Verification items for the finished model (mm, model axes). A direction names the side the tool comes from. Round coordinates to 2 decimals unless told otherwise and drop trailing zeros. Write each loop counter-clockwise with the first axis right and the second up, starting at its lowest first coordinate (ties: lowest second). Pieces come first, ordered by that corner, then holes.
Autodesk Inventor part; units mm, degrees
ref_plane "YZ Plane" through (0, 0, 0) normal (1, 0, 0) x (0, 1, 0)
ref_plane "XZ Plane" through (0, 0, 0) normal (0, 1, 0) x (-1, 0, 0)
ref_plane "XY Plane" through (0, 0, 0) normal (0, 0, 1) x (1, 0, 0)
ref_plane "Work Plane5" through (0, 3, 0) normal (0, 1, 0) x (1, 0, 0)
ref_plane "Work Plane2" through (0, 0, 0) normal (0, -1, 0) x (1, 0, 0)
ref_plane "Work Plane1" through (0, 3, 0) normal (0, 1, 0) x (1, 0, 0)
ref_plane "Work Plane7" through (0, 3, 0) normal (0, -1, 0) x (1, 0, 0)
sketch "Sketch77" plane through (0, 3, 0) normal (0, -1, 0) x (1, 0, 0)
  circle A0 centre (16, 0) radius 17.5
  point P0 (0, 0)
  dimension "d219" = 35
ref_plane "Work Plane6" through (0, 3, 0) normal (0, -1, 0) x (1, 0, 0)
sketch "Sketch78" plane through (0, 3, 0) normal (0, -1, 0) x (1, 0, 0)
  line L0 (45, -30) -> (-13, -30)
  line L1 (-13, -30) -> (-13, 30)
  line L2 (-13, 30) -> (45, 30)
  line L3 (45, 30) -> (45, -30)
  line L4 (45, -30) -> (-13, 30) construction
  line L5 (-13, -30) -> (45, 30) construction
  point P0 (0, 0)
  point P1 (16, 0)
  dimension "d220" = 58
  dimension "d221" = 60
extrude "Extrusion53" add sketch "Sketch78" against normal blind 3
extrude "Extrusion54" cut sketch "Sketch77" against normal blind 3
ref_plane "Work Plane9" through (0, 3, 0) normal (0, -1, 0) x (1, 0, 0)
sketch "Sketch81" plane through (0, 3, 0) normal (0, -1, 0) x (1, 0, 0)
  circle A0 centre (33.5, -25) radius 2.7
  line L0 (-13, -30) -> (45, -30)
  line L1 (45, -30) -> (45, 30)
  circle A1 centre (16, -25) radius 2.7
  circle A2 centre (-1.5, -25) radius 2.7
  circle A3 centre (-6.5, -8) radius 2.7
  circle A4 centre (-6.5, 8) radius 2.7
  circle A5 centre (-1.5, 25) radius 2.7
  circle A6 centre (16, 25) radius 2.7
  circle A7 centre (33.5, 25) radius 2.7
  point P0 (0, 0)
  dimension "mag_D" = 5.4
  dimension "d232" = 5
  dimension "d233" = 11.5
  dimension "d234" = 5.4
  dimension "d235" = 17.5
  dimension "d236" = 5.4
  dimension "d237" = 17.5
  dimension "d238" = 5.4
  dimension "d239" = 5
  dimension "d240" = 17
  dimension "d241" = 5.4
  dimension "d242" = 16
  dimension "d243" = 5.4
  dimension "d244" = 17
  dimension "d245" = 5.4
  dimension "d246" = 17.5
  dimension "d247" = 5.4
  dimension "d248" = 17.5
  dimension "d249" = 5
extrude "Extrusion56" cut sketch "Sketch81" against normal blind 30
ref_plane "Work Plane8" through (0, 3, 0) normal (0, -1, 0) x (1, 0, 0)
sketch "Sketch83" plane through (0, 3, 0) normal (0, -1, 0) x (1, 0, 0)
  circle A0 centre (-6.5, -8) radius 2.7
  line L0 (-9.1417, -2.4) -> (-9.1417, 2.4)
  line L1 (-9.1417, 2.4) -> (-4.9848, 0)
  line L2 (-4.9848, 0) -> (-9.1417, -2.4)
  point P0 (0, 0)
  point P1 (-9.1417, -8.5581)
  point P2 (-7.756, 0)
  dimension "d253" = 4.8
extrude "Extrusion57" add sketch "Sketch83" along normal blind 4.5 contours L0 L1 L2
sketch "Sketch84" plane through (0, 6, 0) normal (0, 1, 0) x (1, 0, 0)
  point P0 (0, 0)
equation "\"d234\" = mag_D"
equation "\"d236\" = mag_D"
equation "\"d237\" = d235"
equation "\"d238\" = mag_D"
equation "\"d241\" = mag_D"
equation "\"d243\" = mag_D"
equation "\"d244\" = d240"
equation "\"d245\" = mag_D"
equation "\"d246\" = d235"
equation "\"d247\" = mag_D"
equation "\"d248\" = d235"
equation "\"d249\" = d239"
properties part number "liquid_port_v03_printtest"
Q1. Depth check by flat-ended pin: P1, Ø7, axis at x = 33.5, z = 25, coming from the -Y side. Enter the tip coordinate at first touch or a pass-through.
Recorded:
P1: stops at y = 3
Q2. Material ranges on line 1 along Z through (x, y) = (16, 3.7); line 2 along Z through (x, y) = (-6.5, 3.7); line 3 along X through (y, z) = (4, 27), recorded low to high.
Recorded:
line 1: z = -30 to -27.7, -22.3 to -17.5, 17.5 to 22.3, 27.7 to 30
line 2: z = -30 to -10.7, -5.3 to 5.3, 10.7 to 30
line 3: x = -13 to -3.31, 0.31 to 14.19, 17.81 to 31.69, 35.31 to 45
Q3. Release check for a two-part mould opening along X. For faces 4 (the flat face through (3, 3, 14)), 5 (the cylindrical face through (-1.851, 4.479, -22.323)), 6 (the flat face through (-13, 4, 0)), 7 (the cylindrical face through (-1.851, 4.479, 27.677)) record: released by +X, released by -X, zero draft, split by the parting line, or undercut.
Recorded:
face 4: zero draft
face 5: undercut
face 6: released by -X
face 7: undercut
Q4. Tool access check on faces 1 (the flat face through (-7.03, 0.78, -1.18)), 2 (the flat face through (-9.142, 1, 0)), 3 (the flat face through (-7.092, 0.781, 1.217)). Record the directions out of +Z, -Z, +X, -X, +Y, -Y that give a thin tool (end or side, any length) a straight path to the whole face; none if there is none.
Recorded:
face 1: -Z, +X, -Y
face 2: +Z, -Z, -X, -Y
face 3: +Z, +X, -Y
Q5. Sectioned sample at B-B (y = 5). Give the number of separate pieces and of enclosed holes in the cut face, plus the area to 3 significant figures.
Recorded:
separate pieces: 1
enclosed holes: 9
area: 2,330 mm2
Q6. Sectioned sample at A-A (z = 25). Enter the section's corners in (x, y), plus the area to 3 significant figures.
Recorded:
outline: (-13, 3) - (-4.2, 3) - (-4.2, 6) - (-13, 6) - close; (1.2, 3) - (13.3, 3) - (13.3, 6) - (1.2, 6) - close; (18.7, 3) - (30.8, 3) - (30.8, 6) - (18.7, 6) - close; (36.2, 3) - (45, 3) - (45, 6) - (36.2, 6) - close
area: 125 mm2
Q7. Sectioned sample at D-D (x = 23). Enter the section's corners in (y, z).
Recorded:
outline: (3, -30) - (6, -30) - (6, -16.04) - (3, -16.04) - close; (3, 16.04) - (6, 16.04) - (6, 30) - (3, 30) - close
Q8. Sectioned sample at C-C (x = 16). Enter the section's corners in (y, z), plus the area to 3 significant figures.
Recorded:
outline: (3, -30) - (6, -30) - (6, -27.7) - (3, -27.7) - close; (3, -22.3) - (6, -22.3) - (6, -17.5) - (3, -17.5) - close; (3, 17.5) - (6, 17.5) - (6, 22.3) - (3, 22.3) - close; (3, 27.7) - (6, 27.7) - (6, 30) - (3, 30) - close
area: 42.6 mm2
